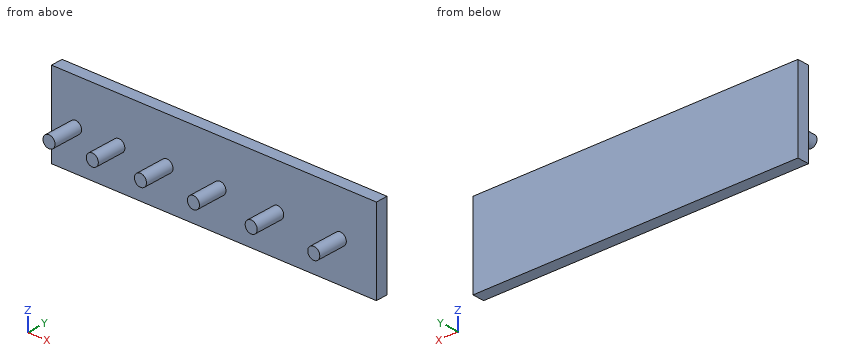
```python
from build123d import *

# Parameters (mm, degrees)
F0_W     = 270
F0_H     = 70
F0_R     = 5
F1_DEPTH = 10
F2_R     = 5
F3_DEPTH = 25


with BuildPart() as f1:
    # F0 (on Front) → F1 (new body)
    with BuildSketch(Plane.XZ):
        with Locations((-11.40806, 1.204433)):
            Rectangle(F0_W, F0_H)
        with Locations((-126.40806, 0)):
            Circle(F0_R, mode=Mode.SUBTRACT)
        with Locations((-90.40806, 0)):
            Circle(F0_R, mode=Mode.SUBTRACT)
        with Locations((-50.40806, 0)):
            Circle(F0_R, mode=Mode.SUBTRACT)
        with Locations((-6.40806, 0)):
            Circle(F0_R, mode=Mode.SUBTRACT)
        with Locations((41.59194, 0)):
            Circle(F0_R, mode=Mode.SUBTRACT)
        with Locations((93.59194, 0)):
            Circle(F0_R, mode=Mode.SUBTRACT)
        with Locations((93.59194, 0)):
            Circle(F0_R)
        with Locations((41.59194, 0)):
            Circle(F0_R)
        with Locations((-6.40806, 0)):
            Circle(F0_R)
        with Locations((-50.40806, 0)):
            Circle(F0_R)
        with Locations((-90.40806, 0)):
            Circle(F0_R)
        with Locations((-126.40806, 0)):
            Circle(F0_R)
    extrude(amount=F1_DEPTH)

    # F2 (on face) → F3 (join)
    with BuildSketch(Plane.XZ.offset(10)):
        with Locations((-126.40806, -0.795567)):
            Circle(F2_R)
        with Locations((-90.40806, -0.795567)):
            Circle(F2_R)
        with Locations((-50.40806, -0.795567)):
            Circle(F2_R)
        with Locations((41.59194, -0.795567)):
            Circle(F2_R)
        with Locations((93.59194, -0.795567)):
            Circle(F2_R)
        with Locations((-6.40806, -0.795567)):
            Circle(F2_R)
    extrude(amount=F3_DEPTH)


solid = f1.part
```
Here's how the part is built. I have some questions about the finished solid (model axes, mm). Coordinates: 2 decimals unless noted, no trailing zeros. Order: outer loops, then holes, each group sorted by start corner. A loop starts at its lowest first (then second) coordinate and runs counter-clockwise, first axis right, second up. Notation, with made-up numbers: M 38,34.25 L 54,34.25 A16 cw 54,51.25 Z; hole C 89.5,86.5 d8. An arc over 180 degrees is marked long. Answer as a JSON object with one key per item and string values. Group by question number.
(1) For pin 1 (8 mm diameter, centred on y = -18.5, z = 5, fed in from +X); pin 2 (8 mm diameter, centred on y = -18, z = 2, fed in from -X), each with a flat end and sliding along its axis, tell me the tip position at first contact or that it passes through.
(2) Suppose I cut it at C-C, the plane z = 9.5. Please give me the cut outline in (x, y).
(3) Suppose I cut it at B-B, the plane x = -90. Please give me the cut outline in (y, z).
(4) I need wall thicknesses on probe 1 along Y at (x, z) = (-22.5, 30); probe 2 along Z at (x, y) = (-9, -17.5); probe 3 along Z at (x, y) = (-4, -32.5). Which ranges of each line are inside material? Lowest first, please.
(5) Suppose I cut it at D-D, the plane x = -127.5. Please give me the cut outline in (y, z).
(6) Suppose I cut it at A-A, the plane y = -26. Please give me the cut outline in (x, z), then the cut area to 3 significant figures.
Values found:
{
 "1": {"pin 1": "stops at x = 98.26", "pin 2": "stops at x = -131.41"},
 "2": {"outline": "M -146.41,-10 L 123.59,-10 L 123.59,0 L -146.41,0 Z"},
 "3": {"outline": "M -35,-5.78 L -10,-5.78 L -10,-33.8 L 0,-33.8 L 0,36.2 L -10,36.2 L -10,4.19 L -35,4.19 Z"},
 "4": {"probe 1": "y = -10 to 0", "probe 2": "z = -5.07 to 3.48", "probe 3": "z = -5.18 to 3.59"},
 "5": {"outline": "M -35,-5.67 L -10,-5.67 L -10,-33.8 L 0,-33.8 L 0,36.2 L -10,36.2 L -10,4.08 L -35,4.08 Z"},
 "6": {"outline": "C -126.41,-0.8 d10; C -90.41,-0.8 d10; C -50.41,-0.8 d10; C -6.41,-0.8 d10; C 41.59,-0.8 d10; C 93.59,-0.8 d10", "area": "471 mm^2"}
}
